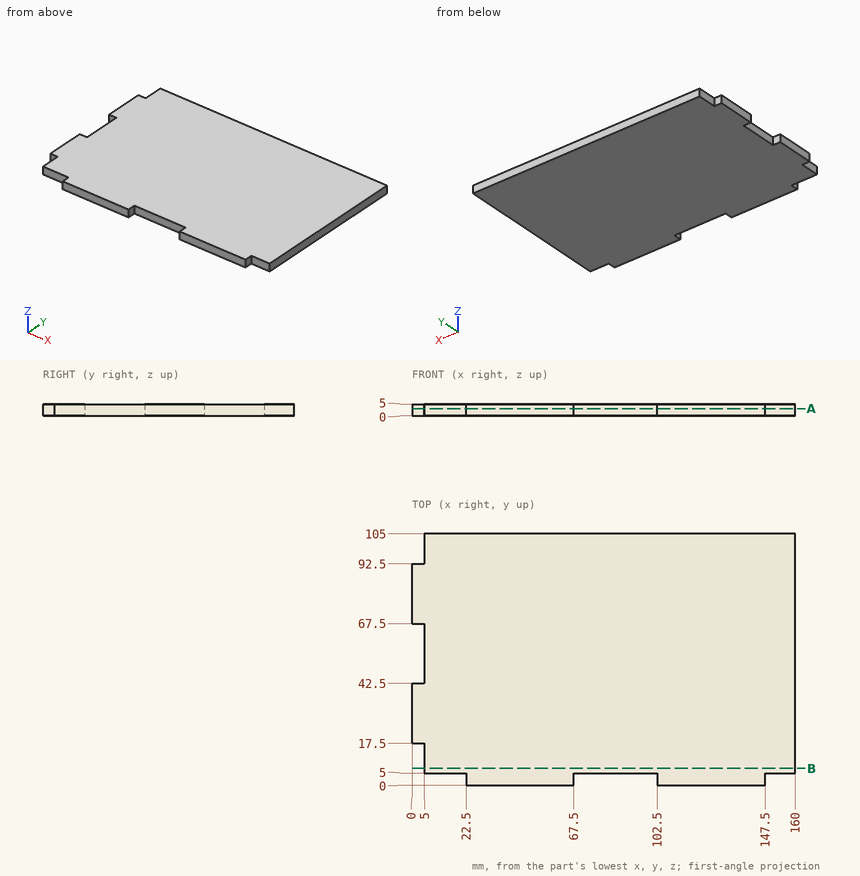
Design review of the part shown in the three views and the two pictorial views. Dimensions are in mm from the part's minimum x, y and z. Round coordinates to 2 decimals unless told otherwise and drop trailing zeros. Write each loop counter-clockwise with the first axis right and the second up, starting at its lowest first coordinate (ties: lowest second). Pieces come first, ordered by that corner, then holes. Notation, with made-up numbers: (11.5, 82) -> (20.5, 82) arc R10 ccw to (20.5, 86) -> close; hole circle Ø11 at (22, 7). An arc over 180 degrees is marked (long way). Write item = value, one per line. Start each with the question number.
1) Wall thickness on probe 1 along X at (y, z) = (60, 1.25); probe 2 along Y at (x, z) = (10, 3): over which ranges is each line inside the solid? List them lowest first. Write a range as from..to.
2) Clearance check with flat-ended pins moving along their axes: pin 1 (2.5 mm diameter, centred on y = 3.5, z = 2, fed in from +X); pin 2 (1.5 mm diameter, centred on x = 83, z = 2.5, fed in from -Y); pin 3 (1.5 mm diameter, centred on x = 3, z = 3.5, fed in from +Y). State where each tip first meets the part, or that it passes through.
3) Take a section at B-B, the plane y = 7. State the section outline as (x, z) points, plus the area to 3 significant figures.
4) Take a section at A-A, the plane z = 3.1. State the section outline as (x, y) points.
Results list:
q1.probe_1 = 5..160
q1.probe_2 = 5..105
q2.pin_1 = 147.5
q2.pin_2 = 5
q2.pin_3 = 92.5
q3.outline = (5, 0) -> (160, 0) -> (160, 5) -> (5, 5) -> close
q3.area = 775 mm²
q4.outline = (0, 17.5) -> (5, 17.5) -> (5, 5) -> (22.5, 5) -> (22.5, 0) -> (67.5, 0) -> (67.5, 5) -> (102.5, 5) -> (102.5, 0) -> (147.5, 0) -> (147.5, 5) -> (160, 5) -> (160, 105) -> (5, 105) -> (5, 92.5) -> (0, 92.5) -> (0, 67.5) -> (5, 67.5) -> (5, 42.5) -> (0, 42.5) -> close
